from build123d import *

# Parameters (mm, degrees)
SKETCH1_R           = 5
SKETCH1_R_2         = 6.5
BOSS_EXTRUDE1_DEPTH = 10


with BuildPart() as part:
    # Sketch1 → Boss-Extrude1 (new body)
    with BuildSketch(Plane.XY):
        with BuildLine():
            Line((14.452049987, 10.106578028), (4.943983372, 10.106578028))
            ThreePointArc((4.943983372, 10.106578028), (1.33240778, 10.781529946), (-1.791639839, 12.715273681))
            ThreePointArc((-1.791639839, 12.715273681), (-23.111525629, 6.446722896), (-7.719583441, -9.58201301))
            ThreePointArc((-7.719583441, -9.58201301), (0.640486438, -11.484150022), (4.454469887, -19.162849381))
            ThreePointArc((4.454469887, -19.162849381), (19.452049987, -33.893421972), (34.449630088, -19.162849381))
            ThreePointArc((34.449630088, -19.162849381), (38.263613537, -11.484150022), (46.623683415, -9.58201301))
            ThreePointArc((46.623683415, -9.58201301), (62.015625604, 6.446722896), (40.695739813, 12.715273681))
            ThreePointArc((40.695739813, 12.715273681), (37.571692195, 10.781529946), (33.960116603, 10.106578028))
            Line((33.960116603, 10.106578028), (24.452049987, 10.106578028))
            Line((24.452049987, 10.106578028), (24.452049987, 17.106578028))
            Line((24.452049987, 17.106578028), (26.952049987, 17.106578028))
            Line((26.952049987, 17.106578028), (23.451304138, 31.692351182))
            Line((23.451304138, 31.692351182), (19.452049987, 31.692351182))
            Line((19.452049987, 31.692351182), (15.452795837, 31.692351182))
            Line((15.452795837, 31.692351182), (11.952049987, 17.106578028))
            Line((11.952049987, 17.106578028), (14.452049987, 17.106578028))
            Line((14.452049987, 17.106578028), (14.452049987, 10.106578028))
        make_face()
        with Locations((-10.547950013, 3.106578028)):
            Circle(SKETCH1_R, mode=Mode.SUBTRACT)
        with Locations((49.452049987, 3.106578028)):
            Circle(SKETCH1_R, mode=Mode.SUBTRACT)
        with Locations((19.452049987, -18.893421972)):
            Circle(SKETCH1_R_2, mode=Mode.SUBTRACT)
    extrude(amount=BOSS_EXTRUDE1_DEPTH)


solid = part.part
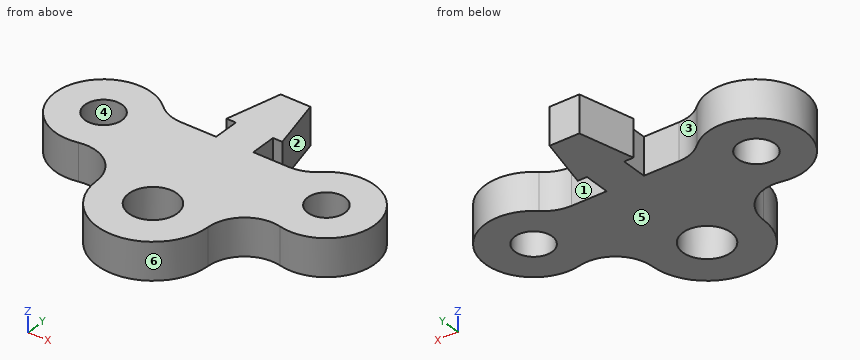
The model under review builds one solid part; all positions refer to its coordinate system, in mm. Face numbers are marked on the shaded views. A direction names the side the tool comes from. Round coordinates to 2 decimals unless told otherwise and drop trailing zeros. Order: outer loops, then holes, each group sorted by start corner. A loop starts at its lowest first (then second) coordinate and runs counter-clockwise, first axis right, second up. Notation, with made-up numbers: (20, -38) -> (61, -38) arc R22 cw to (61, -12) -> close; hole circle Ø5 at (-19, 74.25). An arc over 180 degrees is marked (long way). Write item = value, one per line. Start each with the question number.
Item 1: For line 1 along X through (y, z) = (3, 0.75); line 2 along Y through (x, z) = (49, 3.75); line 3 along X through (y, z) = (7, 5), list the stretches that pass through material, from the lowest coordinate up.
Item 2: Consider section D-D on y = -15.5. Write out the cut boundary in (x, z), plus the area to 3 significant figures.
Item 3: For the marked faces 1, 2 and 3, list the 3-axis set-ups (+Z, -Z, +X, -X, +Y, -Y) from which the entire face can be reached by the end or side of a thin tool; tool diameter is ignored.
Item 4: Consider section A-A on y = 0. Write out the cut boundary in (x, z), plus the area to 3 significant figures.
Item 5: Clearance check with flat-ended pins moving along their axes: pin 1 Ø1.5 at (x, z) = (25.5, 8.5) entering from -Y; pin 2 Ø3 at (x, y) = (40, -14.5) entering from -Z; pin 3 Ø1.5 at (x, z) = (0, 6.5) entering from -Y; pin 4 Ø1.2 at (x, z) = (26, 2.5) entering from -Y. State where each tip first meets the part, or that it passes through.
Item 6: Mouldability with a two-part tool opening along X and no side actions: class the marked faces 4, 5 and 6 as released by +X, released by -X, zero draft, split by the parting line, or undercut.
Item 7: Consider section B-B on z = 8.5. Write out the cut boundary in (x, y), plus the area to 3 significant figures.
Item 8: Consider section C-C on x = 50.5. Write out the cut boundary in (y, z), plus the area to 3 significant figures.
Conclusion:
q1.line_1 = -23.55 to -15.55, -5.55 to 44.45, 54.45 to 62.45
q1.line_2 = -9.89 to -1.87, 8.09 to 16.1
q1.line_3 = -22.95 to -13.69, -7.41 to 46.31, 52.59 to 61.86
q2.outline = (3.69, 0) -> (13.91, 0) -> (13.91, 10) -> (3.69, 10) -> close; (25, 0) -> (35.22, 0) -> (35.22, 10) -> (25, 10) -> close
q2.area = 204 mm2
q3.face_1 = +Z, -Z
q3.face_2 = +Z, -Z, +X, +Y
q3.face_3 = +Z, -Z, +Y
q4.outline = (-23.17, 0) -> (-14.47, 0) -> (-14.47, 10) -> (-23.17, 10) -> close; (-6.63, 0) -> (45.53, 0) -> (45.53, 10) -> (-6.63, 10) -> close; (53.37, 0) -> (62.08, 0) -> (62.08, 10) -> (53.37, 10) -> close
q4.area = 696 mm2
q5.pin_1 = -32.93
q5.pin_2 = through
q5.pin_3 = -11.57
q5.pin_4 = -32.66
q6.face_4 = undercut
q6.face_5 = zero draft
q6.face_6 = split by the parting line
q7.outline = (-7.72, -9.58) arc R10 cw to (4.45, -19.16) arc R15 ccw to (34.45, -19.16) arc R10 cw to (46.62, -9.58) arc R13 ccw (long way) to (40.7, 12.72) arc R10 cw to (33.96, 10.11) -> (24.45, 10.11) -> (24.45, 17.11) -> (26.95, 17.11) -> (23.45, 31.69) -> (15.45, 31.69) -> (11.95, 17.11) -> (14.45, 17.11) -> (14.45, 10.11) -> (4.94, 10.11) arc R10 cw to (-1.79, 12.72) arc R13 ccw (long way) to start; hole circle Ø10 at (-10.55, 3.11); hole circle Ø13 at (19.45, -18.89); hole circle Ø10 at (49.45, 3.11)
q7.area = 2,430 mm2
q8.outline = (-9.85, 0) -> (-1.78, 0) -> (-1.78, 10) -> (-9.85, 10) -> close; (8, 0) -> (16.06, 0) -> (16.06, 10) -> (8, 10) -> close
q8.area = 161 mm2
